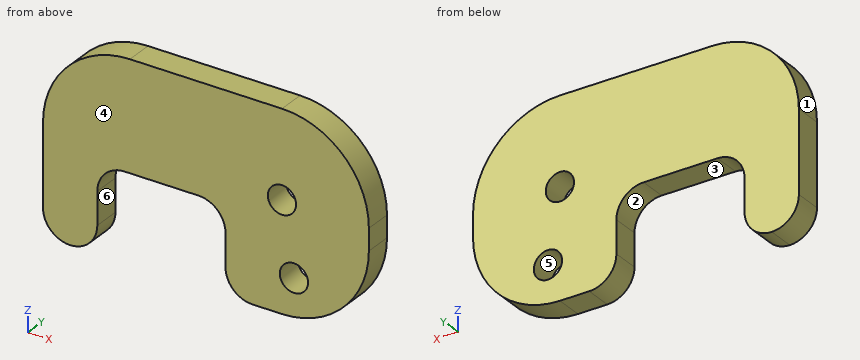
from build123d import *

# Parameters (mm, degrees)
SKETCH1_W           = 38.1
SKETCH1_H           = 22.86
BOSS_EXTRUDE1_DEPTH = 3.175
FILLET1_R           = 10.16
SKETCH3_R           = 1.651
CUT_EXTRUDE1_DEPTH  = 23.44165825
FILLET3_R           = 10.16
SKETCH4_W           = 14.986
SKETCH4_H           = 10.16
CUT_EXTRUDE3_DEPTH  = 23.44165825
FILLET8_R           = 3.175


with BuildPart() as part:
    # Sketch1 → Boss-Extrude1 (new body)
    with BuildSketch(Plane(origin=(0, 0, 0), x_dir=(1, 0, 0), z_dir=(0, 1, 0))):
        Rectangle(SKETCH1_W, SKETCH1_H)
    extrude(amount=BOSS_EXTRUDE1_DEPTH)

    # Fillet1
    fillet1_edges = [part.edges().sort_by_distance(p)[0] for p in [
        (19.05, 1.5875, 11.43),
        (-19.05, 1.5875, 11.43),
    ]]
    fillet(fillet1_edges, radius=FILLET1_R)

    # Sketch3 → Cut-Extrude1 (cut, through all)
    with BuildSketch(Plane(origin=(0, 3.175, 0), x_dir=(1, 0, 0), z_dir=(0, 1, 0))):
        with Locations(Location((8.89, -1.27, 0), (0, 0, 270))):
            Circle(SKETCH3_R)
        with Locations(Location((10.287, 6.994763457, 0), (0, 0, 270))):
            Circle(SKETCH3_R)
    extrude(amount=-CUT_EXTRUDE1_DEPTH, mode=Mode.SUBTRACT)

    # Fillet3
    fillet3_edges = [part.edges().sort_by_distance(p)[0] for p in [
        (19.05, 1.5875, -11.43),
    ]]
    fillet(fillet3_edges, radius=FILLET3_R)

    # Sketch4 → Cut-Extrude3 (cut, through all)
    with BuildSketch(Plane(origin=(0, 3.175, 0), x_dir=(1, 0, 0), z_dir=(0, 1, 0))):
        with Locations((-5.207, 6.35)):
            Rectangle(SKETCH4_W, SKETCH4_H)
    extrude(amount=-CUT_EXTRUDE3_DEPTH, mode=Mode.SUBTRACT)

    # Fillet8
    fillet8_edges = [part.edges().sort_by_distance(p)[0] for p in [
        (-12.7, 1.5875, -1.27),
        (-12.7, 1.5875, -11.43),
        (2.286, 1.5875, -11.43),
        (2.286, 1.5875, -1.27),
        (-19.05, 1.5875, -11.43),
    ]]
    fillet(fillet8_edges, radius=FILLET8_R - 0.0001)  # a hair under: the kernel refuses the full size


solid = part.part
Input: part model. Units: mm. Frame: model coordinates. Face numbers are marked on the shaded views. A direction names the side the tool comes from. Coordinates: 2 decimals unless noted, no trailing zeros. Loops run counter-clockwise (first coordinate to the right, second up) from the corner with the lowest first, then second, coordinate; pieces in that order, holes last. Notation, with made-up numbers: (73.5, -39.5) -> (131.5, -39.5) arc R18 cw to (131.5, -14.5) -> close; hole circle Ø5 at (2, 4.5). An arc over 180 degrees is marked (long way). Write item = value, one per line. Start each with the question number.
Item 1: Reachability of the marked faces 5 and 6 from +Z, -Z, +X, -X, +Y, -Y: full face, straight path, thin tool, end or side. Return the list, or none.
Item 2: Cut plane C-C, the plane x = 8. Return loops of the section in (y, z) (3 decimals), plus the area to 3 significant figures.
Item 3: Mould query, pull axis X, two halves, no side actions, for the marked faces 1, 2, 3 and 4. Classes: pulls with the +X half, pulls with the -X half, needs draft (parallel to the pull), parting line crosses it, or undercut.
Item 4: Cut plane B-B, the plane z = -9.5. Return loops of the section in (x, y) (3 decimals).
Item 5: First-contact query: P1, Ø1.5, axis at y = 2, z = 3.5, coming from the +X side; P2, Ø1.6, axis at y = 2, z = -5.5, coming from the +X side; P3, Ø1.5, axis at y = 2.5, z = 7.5, coming from the -X side. Flat tips, straight axial feed; report the tip coordinate or a pass-through.
Item 6: Cut plane D-D, the plane y = 2. Count the separate pieces of the cut face and the enclosed holes in it, plus the area to 3 significant figures.
Item 7: Material intervals for line 1 (X direction, y = 1.35, z = -8); line 2 (Z direction, x = 9.5, y = 2.65); line 3 (Z direction, x = -4.5, y = 1.3), sorted ascending.
Item 8: Cut plane A-A, the plane z = -6.25. Return loops of the section in (x, y) (3 decimals), plus the area to 3 significant figures.
Ans:
q1.face_5 = +Y, -Y
q1.face_6 = -Z, +Y, -Y
q2.outline = (0, -11.43) -> (3.175, -11.43) -> (3.175, -0.121) -> (0, -0.121) -> close; (0, 2.661) -> (3.175, 2.661) -> (3.175, 11.43) -> (0, 11.43) -> close
q2.area = 63.8 mm²
q3.face_1 = pulls with the -X half
q3.face_2 = undercut
q3.face_3 = undercut
q3.face_4 = needs draft
q4.outline = (-18.796, 0) -> (-12.954, 0) -> (-12.954, 3.175) -> (-18.796, 3.175) -> close; (2.54, 0) -> (14.848, 0) -> (14.848, 3.175) -> (2.54, 3.175) -> close
q5.P1 = 18.94
q5.P2 = 18.45
q5.P3 = -17.45
q6.separate_pieces = 1
q6.enclosed_holes = 2
q6.area = 633 mm²
q7.line_1 = -19.05 to -12.7, 2.29 to 8.98, 11.6 to 16.5
q7.line_2 = -11.41 to -8.45, -5.54 to -0.26, 2.8 to 11.41
q7.line_3 = -1.27 to 11.43
q8.outline = (-19.05, 0) -> (-12.7, 0) -> (-12.7, 3.175) -> (-19.05, 3.175) -> close; (2.286, 0) -> (8.814, 0) -> (8.814, 3.175) -> (2.286, 3.175) -> close; (11.76, 0) -> (17.746, 0) -> (17.746, 3.175) -> (11.76, 3.175) -> close
q8.area = 59.9 mm²
